Part print with two shaded views. Sizes in mm from the minimum x, y, z corner. Coordinates: 2 decimals unless noted, no trailing zeros. Loops run counter-clockwise (first coordinate to the right, second up) from the corner with the lowest first, then second, coordinate; pieces in that order, holes last. Notation, with made-up numbers: (69.25, 37.5) -> (81.25, 37.5) arc R25 ccw to (81.25, 69.5) -> close; hole circle Ø10 at (26, 76.25). An arc over 180 degrees is marked (long way). Return JSON: item names as keys, results as strings. Group by question number.
(1) Probe L1, parallel to Y at x = 11, z = 1.65; L2, parallel to Y at x = 58, z = 1.85; L3, parallel to Y at x = 46, z = 1.25. List the from-to ranges inside material, lowest first.
(2) Saw through at B-B on y = 44.5. Write the cut outline in (x, z).
(3) Saw through at D-D on x = 11. Write the cut outline in (y, z).
(4) Saw through at C-C on z = 3.15. Write the cut outline in (x, y), then the cut area to 3 significant figures.
(5) Saw through at A-A on x = 45.5. Write the cut outline in (y, z), then the cut area to 3 significant figures.
(6) Flat gauge pin, fed straight in: pin 1 Ø2.5 at (x, y) = (58, 4) entering from -Z. Where does the tip first touch, or does it go through?
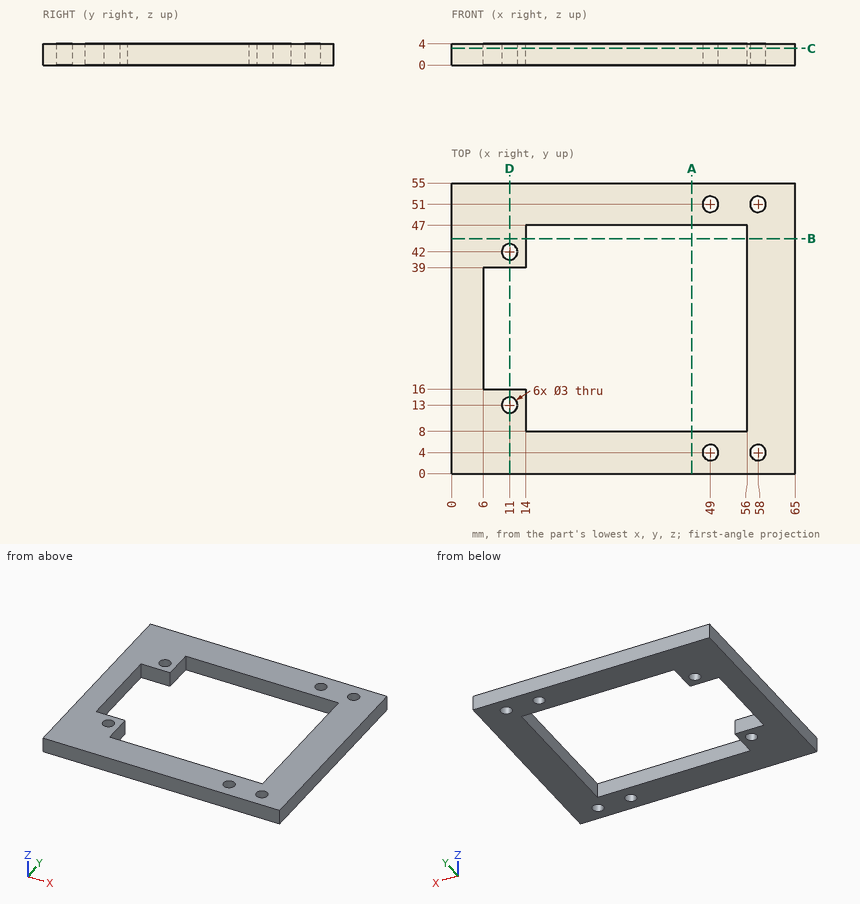
Geometry results:
{
 "1": {"L1": "0 to 11.5, 14.5 to 16, 39 to 40.5, 43.5 to 55", "L2": "0 to 2.5, 5.5 to 49.5, 52.5 to 55", "L3": "0 to 8, 47 to 55"},
 "2": {"outline": "(0, 0) -> (14, 0) -> (14, 4) -> (0, 4) -> close; (56, 0) -> (65, 0) -> (65, 4) -> (56, 4) -> close"},
 "3": {"outline": "(0, 0) -> (11.5, 0) -> (11.5, 4) -> (0, 4) -> close; (14.5, 0) -> (16, 0) -> (16, 4) -> (14.5, 4) -> close; (39, 0) -> (40.5, 0) -> (40.5, 4) -> (39, 4) -> close; (43.5, 0) -> (55, 0) -> (55, 4) -> (43.5, 4) -> close"},
 "4": {"outline": "(0, 0) -> (65, 0) -> (65, 55) -> (0, 55) -> close; hole (6, 16) -> (14, 16) -> (14, 8) -> (56, 8) -> (56, 47) -> (14, 47) -> (14, 39) -> (6, 39) -> close; hole circle Ø3 at (11, 13); hole circle Ø3 at (11, 42); hole circle Ø3 at (49, 4); hole circle Ø3 at (49, 51); hole circle Ø3 at (58, 4); hole circle Ø3 at (58, 51)", "area": "1,710 mm²"},
 "5": {"outline": "(0, 0) -> (8, 0) -> (8, 4) -> (0, 4) -> close; (47, 0) -> (55, 0) -> (55, 4) -> (47, 4) -> close", "area": "64.0 mm²"},
 "6": {"pin 1": "through"}
}
